The listing builds one solid part. Answer for the finished solid, in the listing's coordinates (mm). A direction names the side the tool comes from. Round coordinates to 2 decimals unless told otherwise and drop trailing zeros. Write each loop counter-clockwise with the first axis right and the second up, starting at its lowest first coordinate (ties: lowest second). Pieces come first, ordered by that corner, then holes. Notation, with made-up numbers: (55.5, 49) - (96.5, 49) arc R20 cw to (96.5, 60) - close; hole circle Ø11 at (39, 84). An arc over 180 degrees is marked (long way). Return JSON: item names as keys, results as strings. Group by question number.
(1) Find the intervals of material crossed by line 1 along X through (y, z) = (-5.5, 25); line 2 along X through (y, z) = (-4.25, 4.5); line 3 along X through (y, z) = (-6.25, 3.5), in increasing order. Write a range as [from, to].
(2) Section D-D, the plane y = 6.5 is taken. Write down the section's boundary in (x, z).
(3) Section B-B, the plane z = 15.25 is taken. Write down the section's boundary in (x, y), then the cut area to 3 significant figures.
(4) Section C-C, the plane y = 0 is taken. Write down the section's boundary in (x, z), then the cut area to 3 significant figures.
(5) Which of the six approach directions +Z, -Z, +X, -X, +Y, -Y give full straight-line access (tool end or side, diameter ignored) to faces 1 (the cylindrical face through (-15.632, -7.196, 25.289)), 2 (the cylindrical face through (4.5, -7.5, 3.5)), 3 (the flat face through (0, 0, 7))?
(6) This flat-tipped pin is pushed along its axis until it touches: pin 1 (2 mm diameter, centred on x = -12.5, z = 21.5, fed in from +Y). Where does it stop, or does it pass through?
(7) Determine the mould class of faces 4 (the cylindrical face through (13.5, 0.13, 7.86)), 5 (the flat face through (-0.45, 0, 3)), 6 (the cylindrical face through (15.668, -7.289, 25.196)) for opening direction X: +X half, -X half, draft (parallel to the pull), parting line (faces both ways), or undercut.
(8) Section A-A, the plane x = 4.45 is taken. Write down the section's boundary in (y, z), then the cut area to 3 significant figures.
```python
from build123d import *

# Parameters (mm, degrees)
SKETCH1_W           = 33.8
SKETCH1_H           = 18
BOSS_EXTRUDE1_DEPTH = 7
SKETCH2_W           = 2.5
SKETCH2_H           = 18
BOSS_EXTRUDE2_DEPTH = 20
SKETCH3_R           = 1.4
CUT_EXTRUDE1_DEPTH  = 34.8
FILLET1_R           = 6
FILLET2_R           = 3


with BuildPart() as part:
    # Sketch1 → Boss-Extrude1 (new body)
    with BuildSketch(Plane.XY):
        Rectangle(SKETCH1_W, SKETCH1_H)
        with BuildLine():
            Line((-0.45, 3.5), (-0.45, -3.5))
            ThreePointArc((-0.45, -3.5), (-4.45, -7.5), (-8.45, -3.5))
            Line((-8.45, -3.5), (-8.45, 3.5))
            ThreePointArc((-8.45, 3.5), (-4.45, 7.5), (-0.45, 3.5))
        make_face(mode=Mode.SUBTRACT)
        with BuildLine():
            Line((8.45, 3.5), (8.45, -3.5))
            ThreePointArc((8.45, -3.5), (4.45, -7.5), (0.45, -3.5))
            Line((0.45, -3.5), (0.45, 3.5))
            ThreePointArc((0.45, 3.5), (4.45, 7.5), (8.45, 3.5))
        make_face(mode=Mode.SUBTRACT)
    extrude(amount=BOSS_EXTRUDE1_DEPTH)

    # Sketch2 → Boss-Extrude2 (add)
    with BuildSketch(Plane.XY.offset(7)):
        with Locations((-15.65, 0)):
            Rectangle(SKETCH2_W, SKETCH2_H)
        with Locations((15.65, 0)):
            Rectangle(SKETCH2_W, SKETCH2_H)
    extrude(amount=BOSS_EXTRUDE2_DEPTH)

    # Sketch3 → Cut-Extrude1 (cut, through all)
    with BuildSketch(Plane(origin=(16.9, 0, 0), x_dir=(0, 0, -1), z_dir=(1, 0, 0))):
        with Locations((-24.1, 0)):
            Circle(SKETCH3_R)
    extrude(amount=-CUT_EXTRUDE1_DEPTH, mode=Mode.SUBTRACT)

    # Fillet1
    fillet1_edges = [part.edges().sort_by_distance(p)[0] for p in [
        (15.65, -9, 27),
        (-15.65, -9, 27),
        (-15.65, 9, 27),
        (15.65, 9, 27),
    ]]
    fillet(fillet1_edges, radius=FILLET1_R)

    # Fillet2
    fillet2_edges = [part.edges().sort_by_distance(p)[0] for p in [
        (14.4, 0, 7),
        (-14.4, 0, 7),
    ]]
    fillet(fillet2_edges, radius=FILLET2_R)


solid = part.part
```
Working result:
{
 "1": {"line 1": "x = [-16.9, -14.4], [14.4, 16.9]", "line 2": "x = [-16.9, -8.38], [-0.52, 0.52], [8.38, 16.9]", "line 3": "x = [-16.9, -7.35], [-1.55, 1.55], [7.35, 16.9]"},
 "2": {"outline": "(-16.9, 0) - (-7.1, 0) - (-7.1, 7) - (-11.4, 7) arc R3 cw to (-14.4, 10) - (-14.4, 25.87) - (-16.9, 25.87) - close; (-1.8, 0) - (1.8, 0) - (1.8, 7) - (-1.8, 7) - close; (7.1, 0) - (16.9, 0) - (16.9, 25.87) - (14.4, 25.87) - (14.4, 10) arc R3 cw to (11.4, 7) - (7.1, 7) - close"},
 "3": {"outline": "(-16.9, -9) - (-14.4, -9) - (-14.4, 9) - (-16.9, 9) - close; (14.4, -9) - (16.9, -9) - (16.9, 9) - (14.4, 9) - close", "area": "90.0 mm^2"},
 "4": {"outline": "(-16.9, 0) - (-8.45, 0) - (-8.45, 7) - (-11.4, 7) arc R3 cw to (-14.4, 10) - (-14.4, 22.7) - (-16.9, 22.7) - close; (-16.9, 25.5) - (-14.4, 25.5) - (-14.4, 27) - (-16.9, 27) - close; (-0.45, 0) - (0.45, 0) - (0.45, 7) - (-0.45, 7) - close; (8.45, 0) - (16.9, 0) - (16.9, 22.7) - (14.4, 22.7) - (14.4, 10) arc R3 cw to (11.4, 7) - (8.45, 7) - close; (14.4, 25.5) - (16.9, 25.5) - (16.9, 27) - (14.4, 27) - close", "area": "214 mm^2"},
 "5": {"face 1": "+Z, +X, -X, -Y", "face 2": "+Z, -Z", "face 3": "+Z, +Y, -Y"},
 "6": {"pin 1": "passes through"},
 "7": {"face 4": "undercut", "face 5": "undercut", "face 6": "draft"},
 "8": {"outline": "(-9, 0) - (-7.5, 0) - (-7.5, 7) - (-9, 7) - close; (7.5, 0) - (9, 0) - (9, 7) - (7.5, 7) - close", "area": "21.0 mm^2"}
}
